```python
from build123d import *

# Parameters (mm, degrees)
SKETCH2_R           = 28
BOSS_EXTRUDE1_DEPTH = 60
SKETCH3_R           = 23
CUT_EXTRUDE2_DEPTH  = 72.888803022
CUT_EXTRUDE3_DEPTH  = 72.888803022


with BuildPart() as part:
    # Sketch2 → Boss-Extrude1 (new body)
    with BuildSketch(Plane(origin=(0, 0, 0), x_dir=(1, 0, 0), z_dir=(0, 1, 0))):
        with Locations(Location((0, 0, 0), (0, 0, 270))):
            Circle(SKETCH2_R)
    extrude(amount=BOSS_EXTRUDE1_DEPTH)

    # Sketch3 → Cut-Extrude2 (cut, through all)
    with BuildSketch(Plane.XZ):
        with Locations(Location((0, 0, 0), (0, 0, 270))):
            Circle(SKETCH3_R)
    extrude(amount=-CUT_EXTRUDE2_DEPTH, mode=Mode.SUBTRACT)

    # Sketch5 → Cut-Extrude3 (cut, through all)
    with BuildSketch(Plane.XZ):
        with BuildLine():
            Line((0, 28), (0, 25.5))
            ThreePointArc((0, 25.5), (3.722882581, 25.226774373), (7.365985795, 24.412952572))
            Line((7.365985795, 24.412952572), (6.634014205, 22.022485226))
            ThreePointArc((6.634014205, 22.022485226), (-23.141150891, 0), (6.634014205, -22.022485226))
            Line((6.634014205, -22.022485226), (7.365978971, -24.412930285))
            ThreePointArc((7.365978971, -24.412930285), (3.723999827, -25.234351011), (0, -25.5))
            Line((0, -25.5), (0, -28))
            ThreePointArc((0, -28), (-28, 0), (0, 28))
        make_face()
    extrude(amount=-CUT_EXTRUDE3_DEPTH, mode=Mode.SUBTRACT)


with BuildPart() as body_2:
    # of the pieces the cut leaves, the one that is kept (cut_extrude3_keep)
    add(part.part.solids().sort_by_distance((0, 0, 28))[0])


solid = body_2.part
```
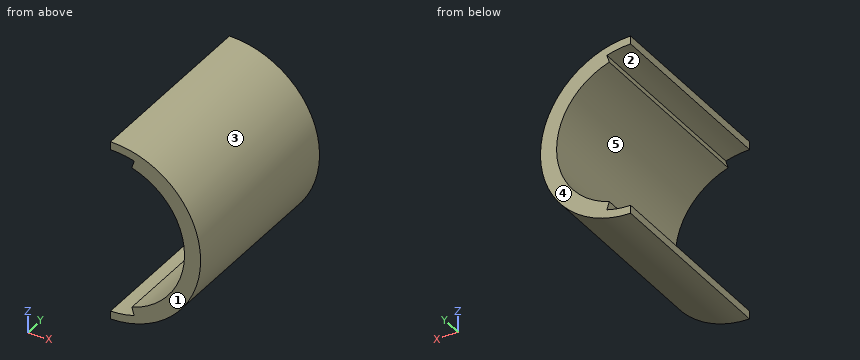
Work out the finished part from the listing and answer in its coordinate system (mm). Face numbers are marked on the shaded views. A direction names the side the tool comes from. Give positions to 0.01 mm unless a question says otherwise; leave off trailing zeros. Order: outer loops, then holes, each group sorted by start corner. A loop starts at its lowest first (then second) coordinate and runs counter-clockwise, first axis right, second up. Notation, with made-up numbers: (-15.5, -34.75) - (-0.5, -34.75) arc R34 ccw to (-0.5, -0.75) - close; hole circle Ø8 at (63, 36). An arc over 180 degrees is marked (long way). One line per item, written item: value. Start each with the question number.
1. Section B-B, the plane y = 16 is taken. Write down the section's boundary in (x, z), then the cut area to 3 significant figures.
2. Section A-A, the plane x = 21 is taken. Write down the section's boundary in (y, z).
3. Consider line 1 (Z direction, x = 13.75, y = 51); line 2 (Z direction, x = 1.5, y = 6); line 3 (X direction, y = 16.5, z = -19.5). Determine where each line is inside the solid, lowest interval first.
4. Which of the six approach directions +Z, -Z, +X, -X, +Y, -Y give full straight-line access (tool end or side, diameter ignored) to the marked faces 1 and 2?
5. Section D-D, the plane x = 26.25 is taken. Write down the section's boundary in (y, z), then the cut area to 3 significant figures.
6. For a pull along Z with two mould halves and no side action, classify the marked faces 3, 4 and 5 as released by +Z, released by -Z, zero draft, split by the parting line, or undercut.
7. Section C-C, the plane z = 0 is taken. Write down the section's boundary in (x, y), then the cut area to 3 significant figures.
8. Each of these flat-tipped pins is pushed along its axis until it touches: pin 1 Ø8 at (y, z) = (17, 5) entering from +X; pin 2 Ø3 at (x, y) = (10.5, 29) entering from +Z; pin 3 Ø2 at (x, y) = (5, 45) entering from +Z. Where does it stop, or does it pass through?
Filled sheet:
1. outline: (0, -28) arc R28 ccw to (0, 28) - (0, 25.5) arc R25.5 cw to (7.37, 24.41) - (6.63, 22.02) arc R23 cw to (6.63, -22.02) - (7.37, -24.41) arc R24.81 cw to (0, -25.5) - close
1. area: 365 mm²
2. outline: (0, -18.52) - (60, -18.52) - (60, -9.38) - (0, -9.38) - close; (0, 9.38) - (60, 9.38) - (60, 18.52) - (0, 18.52) - close
3. line 1: -24.39 to -18.44, 18.44 to 24.39
3. line 2: -27.96 to -25.46, 25.46 to 27.96
3. line 3: 12.2 to 20.09
4. face 1: +Z, -Z, +X, -X, -Y
4. face 2: -X, +Y, -Y
5. outline: (0, -9.74) - (60, -9.74) - (60, 9.74) - (0, 9.74) - close
5. area: 1,170 mm²
6. face 3: split by the parting line
6. face 4: zero draft
6. face 5: undercut
7. outline: (23, 0) - (28, 0) - (28, 60) - (23, 60) - close
7. area: 300 mm²
8. pin 1: x = 27.98
8. pin 2: z = 26.51
8. pin 3: z = 27.71
